Can you work these out from the model? Positions are in its coordinate system, mm. Face numbers are marked on the shaded views. A direction names the side the tool comes from. Round coordinates to 2 decimals unless told otherwise and drop trailing zeros. Write each loop counter-clockwise with the first axis right and the second up, starting at its lowest first coordinate (ties: lowest second). Pieces come first, ordered by that corner, then holes. Notation, with made-up numbers: (79.25, 80) - (124.25, 80) arc R20 ccw to (124.25, 114) - close; hole circle Ø9 at (-30.5, 35.25). An arc over 180 degrees is marked (long way). One line per item, written item: value. Start each with the question number.
(1) I want a section at A-A on x = -25.4. List the corners of the cut face in (y, z) for me (3 decimals).
(2) On a 3-axis mill with a long thin cutter (end or side, diameter ignored), from which of +Z, -Z, +X, -X, +Y, -Y can I reach the whole of each face in a straight line? I mean the marked faces 1, 2 and 3. Say none if no direction works.
(3) I want a section at D-D on x = -114. List the corners of the cut face in (y, z) for me, plus the area to 3 significant figures.
(4) I want a section at C-C on y = 44. List the corners of the cut face in (x, z) for me, plus the area to 3 significant figures.
(5) If I drill on L1, parallel to Y at x = -25.4, z = 7.5 (3 decimals); L2, parallel to Y at x = -92.5, z = 4; L3, parallel to X at y = -36, z = 10, over which ranges is the centre line in solid material (lowest first)? Write a range as from..to.
(6) I'm going to push flat-ended pins straight in: pin 1 Ø17 at (x, y) = (-25.4, 47.625) entering from +Z; pin 2 Ø6.5 at (x, y) = (-25.4, -22.225) entering from +Z; pin 3 Ø1.5 at (x, z) = (-109.5, 15.5) entering from +Y. Where does each tip first touch, or does it pass through?
(7) I want a section at B-B on z = 3. List the corners of the cut face in (x, y) for me (3 decimals).
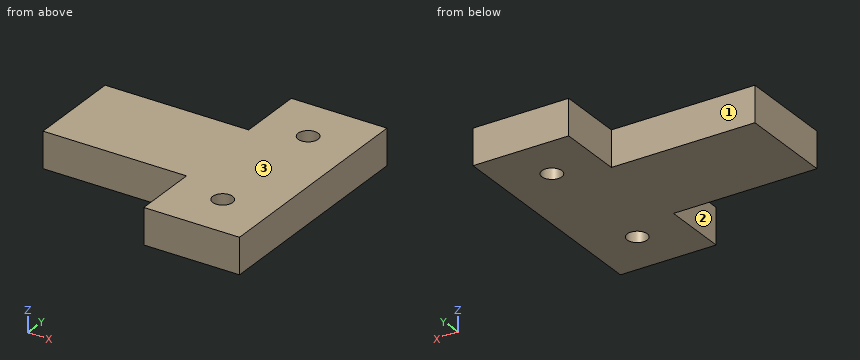
Autodesk Inventor part; units mm, degrees
ref_plane "YZ Plane" through (0, 0, 0) normal (1, 0, 0) x (0, 1, 0)
ref_plane "XZ Plane" through (0, 0, 0) normal (0, 1, 0) x (-1, 0, 0)
ref_plane "XY Plane" through (0, 0, 0) normal (0, 0, 1) x (1, 0, 0)
sketch "Sketch1" plane through (0, 0, 0) normal (0, 0, 1) x (1, 0, 0)
  line L0 (0, 0) -> (-127, 0)
  line L1 (0, 0) -> (0, 25.4)
  line L2 (0, 25.4) -> (-127, 25.4)
  line L3 (-127, 0) -> (-127, 25.4)
  line L4 (0, 73.025) -> (-50.8, 73.025)
  line L5 (-50.8, 73.025) -> (-50.8, -47.625)
  line L6 (-50.8, -47.625) -> (0, -47.625)
  line L7 (0, -47.625) -> (0, 73.025)
  line L8 (-50.8, 38.1) -> (-127, 38.1)
  line L9 (-127, 38.1) -> (-127, -12.7)
  line L10 (-127, -12.7) -> (-50.8, -12.7)
  line L11 (-50.8, -12.7) -> (-50.8, 38.1)
  line L12 (-150.4488, 12.7) -> (41.0315, 12.7)
  dimension "d0" = 50.8
  dimension "d1" = 0
  dimension "d2" = 50.8
  dimension "d4" = 120.65
  dimension "d5" = 60.325
  dimension "d6" = 25.4
extrude "Extrusion1" add sketch "Sketch1" along normal blind 19.05
hole "Hole1" at (-25.4, 47.625, 19.05) direction (0, 0, -1) diameter 10.5918 end through all
hole "Hole2" at (-25.4, -22.225, 19.05) direction (0, 0, -1) diameter 10.5918 end through all
equation "\"d2\" = d0"
equation "\"d5\" = 0.5 * d4"
equation "\"d6\" = 0.5 * d2"
properties part number "Tbracket"
Established:
1. outline: (-47.625, 0) - (-27.521, 0) - (-27.521, 19.05) - (-47.625, 19.05) - close; (-16.929, 0) - (42.329, 0) - (42.329, 19.05) - (-16.929, 19.05) - close; (52.921, 0) - (73.025, 0) - (73.025, 19.05) - (52.921, 19.05) - close
2. face 1: +Z, -Z, -X, +Y
2. face 2: +Z, -Z, -X, -Y
2. face 3: +Z, +X, -X, +Y, -Y
3. outline: (-12.7, 0) - (38.1, 0) - (38.1, 19.05) - (-12.7, 19.05) - close
3. area: 968 mm2
4. outline: (-50.8, 0) - (-29.26, 0) - (-29.26, 19.05) - (-50.8, 19.05) - close; (-21.54, 0) - (0, 0) - (0, 19.05) - (-21.54, 19.05) - close
4. area: 821 mm2
5. L1: -47.625..-27.521, -16.929..42.329, 52.921..73.025
5. L2: -12.7..38.1
5. L3: -50.8..0
6. pin 1: z = 19.05
6. pin 2: through
6. pin 3: y = 38.1
7. outline: (-127, -12.7) - (-50.8, -12.7) - (-50.8, -47.625) - (0, -47.625) - (0, 73.025) - (-50.8, 73.025) - (-50.8, 38.1) - (-127, 38.1) - close; hole circle Ø10.592 at (-25.4, -22.225); hole circle Ø10.592 at (-25.4, 47.625)
